Autodesk Inventor part; units mm, degrees
ref_plane "YZ Plane" through (0, 0, 0) normal (1, 0, 0) x (0, 1, 0)
ref_plane "XZ Plane" through (0, 0, 0) normal (0, 1, 0) x (-1, 0, 0)
ref_plane "XY Plane" through (0, 0, 0) normal (0, 0, 1) x (1, 0, 0)
sketch "Sketch1" plane through (0, 0, 0) normal (1, 0, 0) x (0, 1, 0)
  circle A0 centre (0, 0) radius 12.5
  dimension "d0" = 25
extrude "Extrusion1" add sketch "Sketch1" along normal blind 170
sketch "Sketch2" plane through (170, 0, 0) normal (1, 0, 0) x (0, 0, -1)
  circle A0 centre (0, 0) radius 12.5
  dimension "d3" = 25
extrude "Extrusion2" cut sketch "Sketch2" against normal blind 10
sketch "Sketch3" plane through (160, 0, 0) normal (1, 0, 0) x (0, 0, -1)
  circle A0 centre (0, 0) radius 5
  dimension "d6" = 10
extrude "Extrusion3" add sketch "Sketch3" along normal blind 10
sketch "Sketch4" plane through (0, 0, 0) normal (-1, 0, 0) x (0, 0, 1)
  circle A0 centre (0, 0) radius 12.5
  dimension "d9" = 25
extrude "Extrusion4" cut sketch "Sketch4" against normal blind 10
sketch "Sketch5" plane through (10, 0, 0) normal (-1, 0, 0) x (0, 0, 1)
  circle A0 centre (0, 0) radius 5
  circle A1 centre (0, 0) radius 5
extrude "Extrusion5" add sketch "Sketch5" along normal blind 10
sketch "Sketch6" plane through (170, 0, 0) normal (1, 0, 0) x (0, 0, -1)
  circle A0 centre (0, 0) radius 4
  dimension "d14" = 8
extrude "Extrusion6" cut sketch "Sketch6" against normal blind 170
properties part number "laserbody" material "Polycarbonate, Clear"
Check sheet for the modelled part. Datum: model origin and axes. Units: mm. A direction names the side the tool comes from. Coordinates: 2 decimals unless noted, no trailing zeros. Write each loop counter-clockwise with the first axis right and the second up, starting at its lowest first coordinate (ties: lowest second). Pieces come first, ordered by that corner, then holes.
Item 1: Depth check by flat-ended pin: pin 1 Ø4 at (x, z) = (34.5, 4) entering from -Y; pin 2 Ø1 at (y, z) = (-0.5, 7) entering from -X; pin 3 Ø5 at (x, y) = (101, 3.5) entering from +Z; pin 4 Ø6.5 at (y, z) = (0, 0) entering from -X. Enter the tip coordinate at first touch or a pass-through.
Numbers:
pin 1: stops at y = -12.34
pin 2: stops at x = 10
pin 3: stops at z = 12.46
pin 4: passes through
Item 2: Cross-section at D-D on z = 10. Record the boundary of the cut face in (x, y), then the cut area to 3 significant figures.
Numbers:
outline: (10, -7.5) - (160, -7.5) - (160, 7.5) - (10, 7.5) - close
area: 2,250 mm2
Item 3: Cross-section at C-C on x = 51. Record the boundary of the cut face in (y, z).
Numbers:
outline: circle Ø25 at (0, 0); hole circle Ø8 at (0, 0)
Item 4: Mould release check, pull along Y, two halves, no side actions. Record for faces 1 (the face through (86.19, -3.905, 0.867)), 2 (the face through (164.93, 4.88, 1.08)), 3 (the face through (10, -5.4, -0.2)): released by +Y, released by -Y, zero draft, split by the parting line, or undercut.
Numbers:
face 1: undercut
face 2: split by the parting line
face 3: zero draft
Item 5: Cross-section at A-A on z = 0. Record the boundary of the cut face in (x, y).
Numbers:
outline: (0, -5) - (10, -5) - (10, -12.5) - (160, -12.5) - (160, -5) - (170, -5) - (170, -4) - (0, -4) - close; (0, 4) - (170, 4) - (170, 5) - (160, 5) - (160, 12.5) - (10, 12.5) - (10, 5) - (0, 5) - close
Item 6: Access from +Z, -Z, +X, -X, +Y, -Y to the whole of each face (thin tool, end or side, straight path). Record for faces 4 (the face through (160, -5.4, 0.2)), 5 (the face through (83.95, 11.923, -3.755)), 6 (the face through (5.07, 4.88, -1.08)).
Numbers:
face 4: +X
face 5: +X, -X
face 6: -X
Item 7: Scan lines: probe 1 along Y at (x, z) = (81.5, 0); probe 2 along X at (y, z) = (5.5, 6.25); probe 3 along Z at (x, y) = (90, -1.5). Record each from-to range of solid material in increasing order.
Numbers:
probe 1: y = -12.5 to -4, 4 to 12.5
probe 2: x = 10 to 160
probe 3: z = -12.41 to -3.71, 3.71 to 12.41
